The model under review builds one solid part; all positions refer to its coordinate system, in mm. A direction names the side the tool comes from. Give positions to 0.01 mm unless a question says otherwise; leave off trailing zeros. Order: outer loops, then holes, each group sorted by start corner. A loop starts at its lowest first (then second) coordinate and runs counter-clockwise, first axis right, second up. Notation, with made-up numbers: (56, -9) - (82, -9) arc R11 ccw to (82, -3) - close; hole circle Ø8 at (-5.75, 36.5). An arc over 180 degrees is marked (long way). Write item = value, one per line. Start each with the question number.
1. Machinability: for faces 1 (the cylindrical face through (865.6, 4.77, -29.1)), 2 (the cylindrical face through (890.178, 12.704, -28.924)), which of the approach directions +Z, -Z, +X, -X, +Y, -Y give a long, thin tool a straight path to every point of the face, cutting with its end or side? Answer none if there is none.
2. For P1, Ø12, axis at x = 1221.359, z = -28.575, coming from the +Y side; P2, Ø5, axis at x = 303, y = 21, coming from the +Z side; P3, Ø5, axis at x = 1787.525, z = -28.575, coming from the -Y side, all flat-tipped, find the tip position at first contact; note any pin that passes through.
3. Wall thickness on probe 1 along Z at (x, y) = (868.5, 25.75); probe 2 along Z at (x, y) = (357.5, 26.5); probe 3 along Y at (x, z) = (1448, -25): over which ranges is each line inside the solid? List them lowest first.
4. We need section A-A, the plane y = 24.25. Give the boundary of the cut face in (x, z) (3 decimals), and give its area (3 significant figures).
from build123d import *

# Parameters (mm, degrees)
SKETCH1_W                   = 1803.4
SKETCH1_H                   = 57.15
WOOD_BLOCK_DEPTH            = 28.575
FIPPLE_DEPTH                = 6.35
SKETCH3_R                   = 3.81
FINGER_HOLES_DEPTH          = 1805.531577204
FIPPLE_INSIDE_CHAMFER_DEPTH = 6.35
SKETCH8_W                   = 12.7
SKETCH8_H                   = 6.694937241
FLUE_DEPTH                  = 58.42
SKETCH10_R                  = 3.175
DOWEL_PIN_HOLE_DEPTH        = 15.24
SKETCH6_OUTSIDE_W           = 420.056
SKETCH6_OUTSIDE_H           = 391.481
SKETCH6_OUTSIDE_R           = 23.8125
OUTSIDE_DIAMETER_DEPTH      = 1805.531577205
SKETCH11_W                  = 3.175
SKETCH11_H                  = 6.35


with BuildPart() as part:
    # Sketch1 → wood block (new body)
    with BuildSketch(Plane(origin=(0, 0, 0), x_dir=(1, 0, 0), z_dir=(0, 1, 0))):
        with Locations((901.7, 28.575)):
            Rectangle(SKETCH1_W, SKETCH1_H)
    extrude(amount=WOOD_BLOCK_DEPTH)

    # Sketch2 → Inner Bore (revolve, cut)
    with BuildSketch(Plane.XY.offset(-28.575)):
        with BuildLine():
            Line((1771.65, 28.575), (-15.875, 28.575))
            ThreePointArc((-15.875, 28.575), (-11.225320151, 17.349679849), (0, 12.7))
            Line((0, 12.7), (1755.775, 12.7))
            ThreePointArc((1755.775, 12.7), (1767.000320151, 17.349679849), (1771.65, 28.575))
        make_face()
    revolve(axis=Axis((1771.65, 28.575, -28.575), (-1, 0, 0)), mode=Mode.SUBTRACT)

    # Sketch5 → fipple (cut, symmetric)
    with BuildSketch(Plane.XY.offset(-28.575)):
        Polygon((53.975, 28.575), (53.975, 12.1285), (48.951210809, 0), (53.975, 0), (64.135, 0), (97.457779882, 0), (64.135, 12.1285), (64.135, 28.575), align=None)
    extrude(amount=FIPPLE_DEPTH, both=True, mode=Mode.SUBTRACT)

    # Sketch3 → finger holes (cut, through all)
    with BuildSketch(Plane(origin=(0, 0, 0), x_dir=(1, 0, 0), z_dir=(0, 1, 0))):
        with Locations(Location((1476.629, 28.575, 0), (0, 0, 90))):
            Circle(SKETCH3_R)
        with Locations(Location((1306.449, 28.575, 0), (0, 0, 90))):
            Circle(SKETCH3_R)
        with Locations(Location((1221.359, 28.575, 0), (0, 0, 90))):
            Circle(SKETCH3_R)
    extrude(amount=FINGER_HOLES_DEPTH, mode=Mode.SUBTRACT)

    # Sketch9 → fipple inside chamfer (cut, symmetric)
    with BuildSketch(Plane.XY.offset(-28.575)):
        Polygon((64.135, 12.3825), (84.373651693, 14.153152588), (64.135, 16.801291368), align=None)
    extrude(amount=FIPPLE_INSIDE_CHAMFER_DEPTH, both=True, mode=Mode.SUBTRACT)

    # Sketch8 → flue (cut)
    with BuildSketch(Plane.ZY):
        with Locations((-28.575, 14.842545711)):
            Rectangle(SKETCH8_W, SKETCH8_H)
    extrude(amount=-FLUE_DEPTH, mode=Mode.SUBTRACT)

    # Sketch10 → dowel pin hole (cut)
    with BuildSketch(Plane(origin=(0, 28.575, 0), x_dir=(1, 0, 0), z_dir=(0, 1, 0))):
        with Locations(Location((1787.525, 28.575, 0), (0, 0, 270))):
            Circle(SKETCH10_R)
    extrude(amount=-DOWEL_PIN_HOLE_DEPTH, mode=Mode.SUBTRACT)

    # Sketch6 outside → outside diameter (cut, through all)
    with BuildSketch(Plane.ZY):
        with Locations((-28.575, 14.2875)):
            Rectangle(SKETCH6_OUTSIDE_W, SKETCH6_OUTSIDE_H)
        with Locations((-28.575, 28.575)):
            Circle(SKETCH6_OUTSIDE_R, mode=Mode.SUBTRACT)
    extrude(amount=-OUTSIDE_DIAMETER_DEPTH, mode=Mode.SUBTRACT)

    # Sketch11 → end length locator (revolve, cut)
    with BuildSketch(Plane(origin=(0, 28.575, 0), x_dir=(1, 0, 0), z_dir=(0, 1, 0))):
        with Locations((1757.3625, 7.9375)):
            Rectangle(SKETCH11_W, SKETCH11_H)
    revolve(axis=Axis((0, 28.575, -28.575), (1, 0, 0)), mode=Mode.SUBTRACT)


solid = part.part
Model answer:
q1.face_1 = +X, -X, -Y
q1.face_2 = -X, +Y
q2.P1 = 13.88
q2.P2 = -5.31
q2.P3 = 4.76
q3.probe_1 = -52.22 to -44.2, -12.95 to -4.93
q3.probe_2 = -52.3 to -44.31, -12.84 to -4.85
q3.probe_3 = 5.03 to 13.11
q4.outline = (0, -51.991) - (1755.775, -51.991) - (1755.775, -45.493) - (1758.95, -45.493) - (1758.95, -51.991) - (1803.4, -51.991) - (1803.4, -5.159) - (1758.95, -5.159) - (1758.95, -11.657) - (1755.775, -11.657) - (1755.775, -5.159) - (0, -5.159) - (0, -13.301) - (1755.775, -13.301) arc R15.274 cw to (1755.775, -43.849) - (0, -43.849) - close; hole circle Ø6.35 at (1787.525, -28.575)
q4.area = 30,400 mm2
